Design review of the part built by this model. Coordinates are the model's own, in mm. A direction names the side the tool comes from. Coordinates: 2 decimals unless noted, no trailing zeros. Loops run counter-clockwise (first coordinate to the right, second up) from the corner with the lowest first, then second, coordinate; pieces in that order, holes last. Notation, with made-up numbers: (24, 38.5) -> (66, 38.5) arc R19 ccw to (66, 58.5) -> close; hole circle Ø3 at (-36, -36.75). An arc over 180 degrees is marked (long way). Use one line per item in the form item = value. Start each with the question number.
1. Wall thickness on line 1 (Y direction, x = 4, z = -13.25); line 2 (Y direction, x = 0, z = -9); line 3 (X direction, y = 0, z = -8.75): over which ranges is each line inside the solid? List them lowest first. Write a range as from..to.
2. Consider section B-B (y = 0). State the section outline as (x, z) points, then the cut area to 3 significant figures.
3. Consider section D-D (z = -11). State the section outline as (x, y) points.
4. The part is to be moulded in two halves that separate along X. For faces 4 (the face through (5.723, -1.802, -13.479)), 5 (the face through (0, -15, -15)), 6 (the face through (-8.22, -6.31, -0.36)), say which applies: released by +X, released by -X, zero draft, split by the parting line, or undercut.
5. Machinability: for faces 1 (the face through (-2.4, 2.4, 0)), 2 (the face through (-2.6, 0, -7)), 3 (the face through (0, -12.5, -13.5)), which of the approach directions +Z, -Z, +X, -X, +Y, -Y give a long, thin tool a straight path to every point of the face, cutting with its end or side? Answer none if there is none.
6. Consider section C-C (z = -4). State the section outline as (x, y) points.
7. For pin 1 (6.5 mm diameter, centred on x = 0, y = 0, fed in from -Z); pin 2 (2 mm diameter, centred on y = -2, z = -7, fed in from +X); pin 3 (4 mm diameter, centred on x = 0, y = 0, fed in from -Z); pin 4 (10 mm diameter, centred on x = 0.5, y = 0, fed in from +Z), all flat-tipped, find the tip position at first contact; note any pin that passes through.
8. Consider section A-A (x = 0). State the section outline as (y, z) points, then the cut area to 3 significant figures.
from build123d import *
from build123d.topology import SkipClean

# Parameters (mm, degrees)
BASEMODELSKETCH_R                  = 17.5
BASEMODEL_DEPTH                    = 12
KEYTOOTH_DEPTH                     = 3
PATTERNKEY_COUNT                   = 4
CENTERHOLESUPPORTEXTRUSIONSKETCH_R = 6
CENTERHOLESUPPORTEXTRUSION_DEPTH   = 3
INNERHOLEWITHKEY_DEPTH             = 29.939592257
HOLEFORSPRINGAXLESKETCH_R          = 3.5
HOLEFORSPRINGAXLE_DEPTH            = 3.5
ENCODERKEYEND_R                    = 3.15
ENDOERKEYEND_DEPTH                 = 2
CHAMFER1_SIZE                      = 7.5


with BuildPart() as part:
    # BaseModelSketch → BaseModel (new body)
    with BuildSketch(Plane.XY):
        Circle(BASEMODELSKETCH_R)
    extrude(amount=-BASEMODEL_DEPTH)

    # KeyToothSketch → KeyTooth (add)
    with BuildSketch(Plane(origin=(0, 0, -12), x_dir=(-1, 0, 0), z_dir=(0, 0, -1))):
        with BuildLine():
            ThreePointArc((6.375, -16.297526653), (4.683181341, -13.344473155), (1.407662434, -12.420486563))
            ThreePointArc((1.407662434, -12.420486563), (0, -12.5), (-1.407662434, -12.420486563))
            ThreePointArc((-1.407662434, -12.420486563), (-4.683181341, -13.344473155), (-6.375, -16.297526653))
            ThreePointArc((-6.375, -16.297526653), (0, -17.5), (6.375, -16.297526653))
        make_face()
    keytooth = extrude(amount=KEYTOOTH_DEPTH)

    # PatternKey: KeyTooth ×4 about axis
    with SkipClean():  # the faces are left unmerged after this step: merging them gives an invalid solid
        patternkey_axis = Axis((0, 0, 0), (0, 0, 1))
        for i in range(1, PATTERNKEY_COUNT):
            add(keytooth.rotate(patternkey_axis, i * 360 / PATTERNKEY_COUNT))

    # CenterHoleSupportExtrusionSketch → CenterHoleSupportExtrusion (add)
    with SkipClean():  # the faces are left unmerged after this step: merging them gives an invalid solid
        with BuildSketch(Plane(origin=(0, 0, -12), x_dir=(-1, 0, 0), z_dir=(0, 0, -1))):
            with Locations(Location((0, 0, 0), (0, 0, 180))):
                Circle(CENTERHOLESUPPORTEXTRUSIONSKETCH_R)
        extrude(amount=CENTERHOLESUPPORTEXTRUSION_DEPTH)

    # InnerHoleWithKeySketch → InnerHoleWithKey (cut, through all)
    with SkipClean():  # the faces are left unmerged after this step: merging them gives an invalid solid
        with BuildSketch(Plane.XY):
            with BuildLine():
                Line((-2.6, 1.778341924), (-2.6, -1.778341924))
                ThreePointArc((-2.6, -1.778341924), (3.15, 0), (-2.6, 1.778341924))
            make_face()
        extrude(amount=-INNERHOLEWITHKEY_DEPTH, mode=Mode.SUBTRACT)

    # HoleforSpringAxleSketch → HoleforSpringAxle (cut)
    with SkipClean():  # the faces are left unmerged after this step: merging them gives an invalid solid
        with BuildSketch(Plane(origin=(0, 0, -15), x_dir=(-1, 0, 0), z_dir=(0, 0, -1))):
            Circle(HOLEFORSPRINGAXLESKETCH_R)
        extrude(amount=-HOLEFORSPRINGAXLE_DEPTH, mode=Mode.SUBTRACT)

    # EncoderKeyEnd → EndoerKeyEnd (cut)
    with SkipClean():  # the faces are left unmerged after this step: merging them gives an invalid solid
        with BuildSketch(Plane.XY):
            Circle(ENCODERKEYEND_R)
        extrude(amount=-ENDOERKEYEND_DEPTH, mode=Mode.SUBTRACT)

    # Chamfer1
    chamfer1_edges = [part.edges().sort_by_distance(p)[0] for p in [
        (-17.5, 0, 0),
    ]]
    chamfer(chamfer1_edges, length=CHAMFER1_SIZE)


solid = part.part
Geometry check:
q1.line_1 = -17.04..-12.9, -4.47..4.47, 12.9..17.04
q1.line_2 = -17.5..-3.15, 3.15..17.5
q1.line_3 = -17.5..-2.6, 3.15..17.5
q2.outline = (-17.5, -15) -> (-12.5, -15) -> (-12.5, -12) -> (-6, -12) -> (-6, -15) -> (-3.5, -15) -> (-3.5, -11.5) -> (-2.6, -11.5) -> (-2.6, -2) -> (-3.15, -2) -> (-3.15, 0) -> (-10, 0) -> (-17.5, -7.5) -> close; (3.15, -11.5) -> (3.5, -11.5) -> (3.5, -15) -> (6, -15) -> (6, -12) -> (12.5, -12) -> (12.5, -15) -> (17.5, -15) -> (17.5, -7.5) -> (10, 0) -> (3.15, 0) -> close
q2.area = 338 mm²
q3.outline = circle Ø35 at (0, 0); hole (-2.6, -1.78) arc R3.15 ccw (long way) to (-2.6, 1.78) -> close
q4.face_4 = undercut
q4.face_5 = zero draft
q4.face_6 = split by the parting line
q5.face_1 = +Z, +X, -X, +Y, -Y
q5.face_2 = +Z, -Z
q5.face_3 = -Z
q6.outline = circle Ø28 at (0, 0); hole (-2.6, -1.78) arc R3.15 ccw (long way) to (-2.6, 1.78) -> close
q7.pin_1 = -11.5
q7.pin_2 = 17.46
q7.pin_3 = through
q7.pin_4 = 0
q8.outline = (-17.5, -15) -> (-12.5, -15) -> (-12.5, -12) -> (-6, -12) -> (-6, -15) -> (-3.5, -15) -> (-3.5, -11.5) -> (-3.15, -11.5) -> (-3.15, 0) -> (-10, 0) -> (-17.5, -7.5) -> close; (3.15, -11.5) -> (3.5, -11.5) -> (3.5, -15) -> (6, -15) -> (6, -12) -> (12.5, -12) -> (12.5, -15) -> (17.5, -15) -> (17.5, -7.5) -> (10, 0) -> (3.15, 0) -> close
q8.area = 333 mm²
